The listing builds one solid part. Answer for the finished solid, in the listing's coordinates (mm). A direction names the side the tool comes from. Coordinates: 2 decimals unless noted, no trailing zeros. Order: outer loops, then holes, each group sorted by start corner. A loop starts at its lowest first (then second) coordinate and runs counter-clockwise, first axis right, second up. Notation, with made-up numbers: M 38.25,73 L 97.25,73 A27 ccw 97.25,93 Z; hole C 33.5,32.25 d8. An arc over 180 degrees is marked long. One line per item, written item: value. Start each with the question number.
Q1. The part is cut by section B-B on x = 0. Give the vertices of the cut face in (y, z).
Q2. Each of these flat-tipped pins is pushed along its axis until it touches: pin 1 Ø10 at (y, z) = (-3, 7) entering from -X; pin 2 Ø2 at (x, z) = (-5.5, 6.5) entering from -Y; pin 3 Ø2 at (y, z) = (-5.5, 17) entering from +X; pin 4 Ø1.5 at (x, z) = (3, 8.5) entering from +Y. Where does it stop, or does it pass through?
Q3. The part is cut by section A-A on z = 5.5. Give the vertices of the cut face in (x, y), then the cut area to 4 significant figures.
Q4. For faces 1 (the flat face through (5, -5, 0)), 2 (the flat face through (-5.66, -3.2, 7.4)), determine the directions among +Z, -Z, +X, -X, +Y, -Y from which every point of the face is accessible in a straight line to the end or side of a thin tool.
Q5. Straight lines are drawn through the part: line 1 along Z through (x, y) = (-2.5, -5.5); line 2 along Y through (x, z) = (0, 6.75); line 3 along Y through (x, z) = (-7, 4.5). For each, find the intervals that lie inside material, in ascending order. Write a range as [from, to].
Q6. The part is cut by section C-C on z = 16.25. Give the vertices of the cut face in (x, y).
Q7. Determine the mould class of faces 3 (the flat face through (5.66, 3.2, 7.4)), 4 (the cylindrical face through (-14.985, 0.66, 11.128)), 5 (the flat face through (0, 0, 15)), 6 (the flat face through (0, 0, 25)) for opening direction X: pulls with the +X half, pulls with the -X half, needs draft (parallel to the pull), parting line crosses it, or undercut.
```python
from build123d import *

# Parameters (mm, degrees)
F0_R     = 15
F1_DEPTH = 25
F2_R     = 5
F3_R     = 2.5
F4_DEPTH = 15


with BuildPart() as f1:
    # F0 (on Top) → F1 (new body)
    with BuildSketch(Plane.XY):
        Circle(F0_R)
        Polygon((-7.505553, 0), (-3.752777, 6.5), (3.752777, 6.5), (7.505553, 0), (3.752777, -6.5), (-3.752777, -6.5), align=None, mode=Mode.SUBTRACT)
        Polygon((3.752777, 6.5), (-3.752777, 6.5), (-7.505553, 0), (-3.752777, -6.5), (3.752777, -6.5), (7.505553, 0), align=None)
    extrude(amount=F1_DEPTH)

    # F2
    f2_edges = [f1.edges().sort_by_distance(p)[0] for p in [
        (-15, 0, 25),
    ]]
    fillet(f2_edges, radius=F2_R)

    # F3
    f3_edges = [f1.edges().sort_by_distance(p)[0] for p in [
        (-15, 0, 0),
    ]]
    fillet(f3_edges, radius=F3_R)

    # F0 (on Top) → F4 (cut)
    with BuildSketch(Plane.XY):
        Polygon((3.752777, 6.5), (-3.752777, 6.5), (-7.505553, 0), (-3.752777, -6.5), (3.752777, -6.5), (7.505553, 0), align=None)
    extrude(amount=F4_DEPTH, mode=Mode.SUBTRACT)


solid = f1.part
```
Output:
1. outline: M -15,2.5 A2.5 ccw -12.5,0 L -6.5,0 L -6.5,15 L 6.5,15 L 6.5,0 L 12.5,0 A2.5 ccw 15,2.5 L 15,20 A5 ccw 10,25 L -10,25 A5 ccw -15,20 Z
2. pin 1: stops at x = -15
2. pin 2: stops at y = -14.31
2. pin 3: stops at x = 14.31
2. pin 4: stops at y = 14.83
3. outline: C 0,0 d30; hole M -7.51,0 L -3.75,-6.5 L 3.75,-6.5 L 7.51,0 L 3.75,6.5 L -3.75,6.5 Z
3. area: 560.5 mm^2
4. face 1: -Z, +X, -X, +Y, -Y
4. face 2: -Z
5. line 1: z = [15, 25]
5. line 2: y = [-15, -6.5], [6.5, 15]
5. line 3: y = [-13.27, -0.88], [0.88, 13.27]
6. outline: C 0,0 d30
7. face 3: undercut
7. face 4: parting line crosses it
7. face 5: undercut
7. face 6: needs draft
